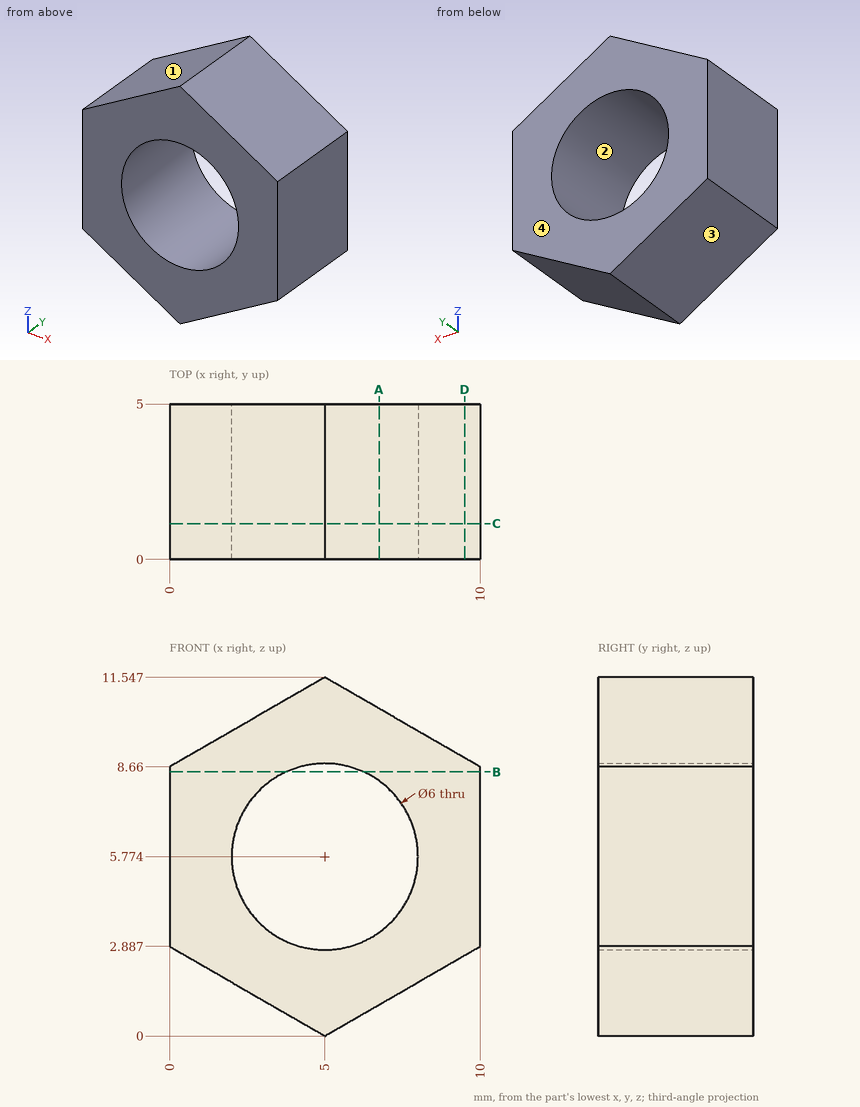
Answer from the drawing. Dimensions are ordinates in mm from the lowest x, y and z of the part. Coordinates: 2 decimals unless noted, no trailing zeros. Order: outer loops, then holes, each group sorted by start corner. A loop starts at its lowest first (then second) coordinate and runs counter-clockwise, first axis right, second up. Notation, with made-up numbers: (86.25, 13.25) - (110.25, 13.25) arc R12 ccw to (110.25, 28.25) - close; hole circle Ø5 at (-6, -26.5). An arc over 180 degrees is marked (long way). Put each result on its own line as item: value. Start each with the question number.
1) Find section A-A (x = 6.75). Give the vertices of the cut face in (y, z).
2) Find section B-B (z = 8.5). Give the vertices of the cut face in (x, y).
3) Find section D-D (x = 9.5). Give the vertices of the cut face in (y, z).
4) For a pull along Z with two mould halves and no side action, classify the marked faces 1, 2, 3 and 4 as released by +Z, released by -Z, zero draft, split by the parting line, or undercut.
5) Find the intervals of material crossed by line 1 (X direction, y = 4.3, z = 4.5) (1 decimal); line 2 (Z direction, x = 3.75, y = 2) (1 decimal); line 3 (X direction, y = 1.35, z = 8.25) (1 decimal), in increasing order. Write a range as from..to.
6) Find section C-C (y = 1.15). Give the vertices of the cut face in (x, z).
Results list:
1. outline: (0, 1.01) - (5, 1.01) - (5, 3.34) - (0, 3.34) - close; (0, 8.21) - (5, 8.21) - (5, 10.54) - (0, 10.54) - close
2. outline: (0, 0) - (3.75, 0) - (3.75, 5) - (0, 5) - close; (6.25, 0) - (10, 0) - (10, 5) - (6.25, 5) - close
3. outline: (0, 2.6) - (5, 2.6) - (5, 8.95) - (0, 8.95) - close
4. face 1: released by +Z
4. face 2: undercut
4. face 3: released by -Z
4. face 4: zero draft
5. line 1: x = 0..2.3, 7.7..10
5. line 2: z = 0.7..3, 8.5..10.8
5. line 3: x = 0..3.3, 6.7..10
6. outline: (0, 2.89) - (5, 0) - (10, 2.89) - (10, 8.66) - (5, 11.55) - (0, 8.66) - close; hole circle Ø6 at (5, 5.77)
